```python
from build123d import *

# Parameters (mm, degrees)
BOSS_EXTRUDE1_DEPTH = 20
SKETCH2_R           = 3.5
CUT_EXTRUDE1_DEPTH  = 4.5
SKETCH3_R           = 3.5
CUT_EXTRUDE2_DEPTH  = 4.5
SKETCH4_W           = 22.25
SKETCH4_H           = 20
CUT_EXTRUDE3_DEPTH  = 4.5
SKETCH5_W           = 20
SKETCH5_H           = 22.25
CUT_EXTRUDE4_DEPTH  = 4.5


with BuildPart() as part:
    # Sketch1 → Boss-Extrude1 (new body)
    with BuildSketch(Plane.XY):
        with BuildLine():
            Line((0, 2), (0, 50))
            Line((0, 50), (3.5, 50))
            Line((3.5, 50), (3.5, 5.5))
            ThreePointArc((3.5, 5.5), (4.085786438, 4.085786438), (5.5, 3.5))
            Line((5.5, 3.5), (50, 3.5))
            Line((50, 3.5), (50, 0))
            Line((50, 0), (2, 0))
            ThreePointArc((2, 0), (0.585786438, 0.585786438), (0, 2))
        make_face()
    extrude(amount=BOSS_EXTRUDE1_DEPTH)

    # Sketch2 → Cut-Extrude1 (cut, through all)
    with BuildSketch(Plane(origin=(0, 3.5, 0), x_dir=(1, 0, 0), z_dir=(0, 1, 0))):
        with Locations((38, -10)):
            Circle(SKETCH2_R)
        with Locations((18, -10)):
            Circle(SKETCH2_R)
    extrude(amount=-CUT_EXTRUDE1_DEPTH, mode=Mode.SUBTRACT)

    # Sketch3 → Cut-Extrude2 (cut, through all)
    with BuildSketch(Plane(origin=(3.5, 0, 0), x_dir=(0, 0, -1), z_dir=(1, 0, 0))):
        with Locations((-10, 38)):
            Circle(SKETCH3_R)
        with Locations((-10, 18)):
            Circle(SKETCH3_R)
    extrude(amount=-CUT_EXTRUDE2_DEPTH, mode=Mode.SUBTRACT)

    # Sketch4 → Cut-Extrude3 (cut, through all)
    with BuildSketch(Plane(origin=(0, 3.5, 0), x_dir=(1, 0, 0), z_dir=(0, 1, 0))):
        with Locations((38.875, -10)):
            Rectangle(SKETCH4_W, SKETCH4_H)
    extrude(amount=-CUT_EXTRUDE3_DEPTH, mode=Mode.SUBTRACT)

    # Sketch5 → Cut-Extrude4 (cut, through all)
    with BuildSketch(Plane(origin=(3.5, 0, 0), x_dir=(0, 0, -1), z_dir=(1, 0, 0))):
        with Locations((-10, 38.875)):
            Rectangle(SKETCH5_W, SKETCH5_H)
    extrude(amount=-CUT_EXTRUDE4_DEPTH, mode=Mode.SUBTRACT)


solid = part.part
```
Here's how the part is built. I have some questions about the finished solid (model axes, mm). A direction names the side the tool comes from. Coordinates: 2 decimals unless noted, no trailing zeros. Order: outer loops, then holes, each group sorted by start corner. A loop starts at its lowest first (then second) coordinate and runs counter-clockwise, first axis right, second up. Notation, with made-up numbers: (12.5, 42) - (58.5, 42) arc R20 ccw to (58.5, 74) - close; hole circle Ø3 at (87, -23). An arc over 180 degrees is marked (long way). One line per question, with ' | ' between items. Start each with the question number.
1. If we section it at D-D (z = 2): Write out the boundary of the cut face in (x, y).
2. Which directions (+Z, -Z, +X, -X, +Y, -Y) give clear straight access to the entire face, cutting with the end or side of a thin tool? Please do faces 1 (the flat face through (27.75, 2, 10)), 2 (the flat face through (3.5, 14, 10)).
3. I'm going to push flat-ended pins straight in: pin 1 Ø5.5 at (x, z) = (18, 10) entering from +Y; pin 2 Ø6 at (x, z) = (13.5, 9.5) entering from +Y; pin 3 Ø2 at (x, z) = (6, 10.5) entering from +Y; pin 4 Ø2 at (x, z) = (21, 12.5) entering from -Y. Where does each tip first touch, or does it pass through?
4. If we section it at B-B (z = 10): Write out the boundary of the cut face in (x, y), and give its area (3 significant figures).
5. If we section it at A-A (y = 18): Write out the boundary of the cut face in (x, z).
6. Please list where these lines run through material, in increasing order: line 1 along Z through (x, y) = (18, 1.55); line 2 along Y through (x, z) = (12, 17.25). Write a range as [from, to].
7. If we mould it in two halves opening along Y, with no side actions, what happens to faces 3 (the cylindrical face through (1.77, 21.47, 10.46)), 4 (the cylindrical face through (0.6, 0.57, 9.86)), 5 (the cylindrical face through (4.07, 4.1, 9.86)), 6 (the flat face through (7, 3, 20))? For each: released by +Y, released by -Y, zero draft, split by the parting line, or undercut.
Model answer:
1) outline: (0, 2) arc R2 ccw to (2, 0) - (27.75, 0) - (27.75, 3.5) - (5.5, 3.5) arc R2 cw to (3.5, 5.5) - (3.5, 27.75) - (0, 27.75) - close
2) face 1: +Z, -Z, +X, +Y, -Y | face 2: +Z, -Z, +X, +Y
3) pin 1: passes through | pin 2: stops at y = 3.5 | pin 3: stops at y = 3.56 | pin 4: stops at y = 0
4) outline: (0, 2) arc R2 ccw to (2, 0) - (14.5, 0) - (14.5, 3.5) - (5.5, 3.5) arc R2 cw to (3.5, 5.5) - (3.5, 14.5) - (0, 14.5) - close; (0, 21.5) - (3.5, 21.5) - (3.5, 27.75) - (0, 27.75) - close; (21.5, 0) - (27.75, 0) - (27.75, 3.5) - (21.5, 3.5) - close | area: 133 mm²
5) outline: (0, 0) - (3.5, 0) - (3.5, 6.5) - (0, 6.5) - close; (0, 13.5) - (3.5, 13.5) - (3.5, 20) - (0, 20) - close
6) line 1: z = [0, 6.5], [13.5, 20] | line 2: y = [0, 3.5]
7) face 3: undercut | face 4: released by -Y | face 5: released by +Y | face 6: zero draft
